Geometry: see drawing. Coordinates: mm, zero at the bounding-box minimum. Coordinates: 2 decimals unless noted, no trailing zeros. Write each loop counter-clockwise with the first axis right and the second up, starting at its lowest first coordinate (ties: lowest second). Pieces come first, ordered by that corner, then holes. Notation, with made-up numbers: (67, 20.25) -> (84, 20.25) arc R11 cw to (84, 24.25) -> close; hole circle Ø9 at (24.5, -29.75). An arc over 180 degrees is marked (long way). Use one line per item in the form item = value. Start each with the question number.
(1) Cut plane A-A on x = 50.8. Return the cut outline in (y, z) (3 decimals), plus the area to 3 significant figures.
(2) First-contact query: pin 1 (23 mm diameter, centred on x = 838.2, z = 57.15, fed in from +Y); pin 2 (17 mm diameter, centred on x = 49, z = 51.5, fed in from -Y) (3 decimals). Flat tips, straight axial feed; report the tip coordinate or a pass-through.
(3) Cut plane B-B on z = 57.15. Return the cut outline in (x, y) (3 decimals), plus the area to 3 significant figures.
(4) Ray query, line 1 along Z through (x, y) = (838.2, 15.25); line 2 along Z through (x, y) = (838.2, 3.25) (3 decimals); line 3 along X through (y, z) = (4, 61). Return the intervals inside material, ascending.
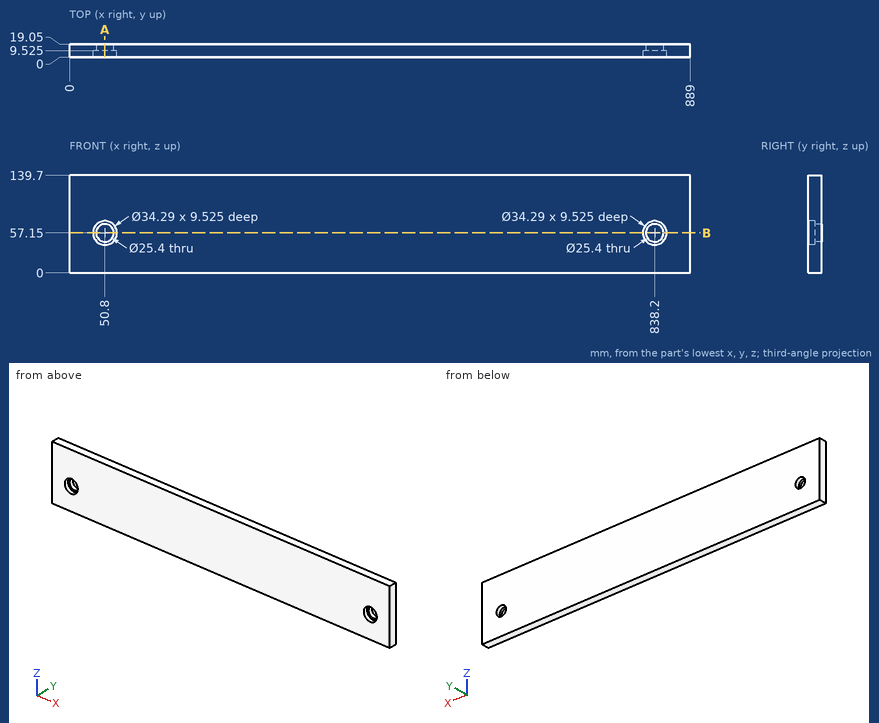
Values:
q1.outline = (0, 0) -> (19.05, 0) -> (19.05, 44.45) -> (9.525, 44.45) -> (9.525, 40.005) -> (0, 40.005) -> close; (0, 74.295) -> (9.525, 74.295) -> (9.525, 69.85) -> (19.05, 69.85) -> (19.05, 139.7) -> (0, 139.7) -> close
q1.area = 2,090 mm2
q2.pin_1 = through
q2.pin_2 = 9.525
q3.outline = (0, 0) -> (33.655, 0) -> (33.655, 9.525) -> (38.1, 9.525) -> (38.1, 19.05) -> (0, 19.05) -> close; (63.5, 9.525) -> (67.945, 9.525) -> (67.945, 0) -> (821.055, 0) -> (821.055, 9.525) -> (825.5, 9.525) -> (825.5, 19.05) -> (63.5, 19.05) -> close; (850.9, 9.525) -> (855.345, 9.525) -> (855.345, 0) -> (889, 0) -> (889, 19.05) -> (850.9, 19.05) -> close
q3.area = 15,800 mm2
q4.line_1 = 0 to 44.45, 69.85 to 139.7
q4.line_2 = 0 to 40.005, 74.295 to 139.7
q4.line_3 = 0 to 34.09, 67.51 to 821.49, 854.91 to 889
